from build123d import *

# Parameters (mm, degrees)
CROQUIS2_W              = 43
CROQUIS2_H              = 82
SALIENTE_EXTRUIR1_DEPTH = 24
CROQUIS3_W              = 24.22772491
CROQUIS3_H              = 79.582021813
CORTAR_EXTRUIR1_DEPTH   = 16
CROQUIS4_W              = 16.121738507
CROQUIS4_H              = 21.293525096
CORTAR_EXTRUIR2_DEPTH   = 10
CORTAR_EXTRUIR4_DEPTH   = 89.103632161
REDONDEO1_R             = 10
SALIENTE_EXTRUIR3_DEPTH = 16
CROQUIS8_W              = 4.909457408
CROQUIS8_H              = 15
SALIENTE_EXTRUIR4_DEPTH = 10
CORTAR_EXTRUIR5_START   = -4.909458
CROQUIS9_R              = 3
CORTAR_EXTRUIR5_DEPTH   = 4.909458
SALIENTE_EXTRUIR5_DEPTH = 9.5
CROQUIS12_W             = 8.494170986
CROQUIS12_H             = 20
SALIENTE_EXTRUIR6_DEPTH = 18
CROQUIS12_3_W           = 8.498446764
CROQUIS12_3_H           = 21
CORTAR_EXTRUIR6_DEPTH   = 15
CROQUIS13_W             = 4.947680971
CROQUIS13_H             = 17.318298189
CORTAR_EXTRUIR8_DEPTH   = 15
REDONDEO6_R             = 4
CROQUIS14_W             = 12
CROQUIS14_H             = 10
SALIENTE_EXTRUIR7_DEPTH = 15
CROQUIS16_R             = 3.3
CORTAR_EXTRUIR9_DEPTH   = 85.026241651
SALIENTE_EXTRUIR8_DEPTH = 10
CROQUIS21_R             = 3.3
CORTAR_EXTRUIR10_DEPTH  = 93.393365129
CROQUIS22_W             = 6
CROQUIS22_H             = 15
SALIENTE_EXTRUIR9_DEPTH = 10
CROQUIS23_R             = 3
CORTAR_EXTRUIR11_DEPTH  = 10


with BuildPart() as part:
    # Croquis2 → Saliente-Extruir1 (new body)
    with BuildSketch(Plane(origin=(0, 0, 0), x_dir=(0, 0, -1), z_dir=(1, 0, 0))):
        Rectangle(CROQUIS2_W, CROQUIS2_H)
    extrude(amount=SALIENTE_EXTRUIR1_DEPTH)

    # Croquis3 → Cortar-Extruir1 (cut)
    with BuildSketch(Plane.ZY):
        with Locations((-6.735600962, -1.208989093)):
            Rectangle(CROQUIS3_W, CROQUIS3_H)
    extrude(amount=-CORTAR_EXTRUIR1_DEPTH, mode=Mode.SUBTRACT)

    # Croquis4 → Cortar-Extruir2 (cut)
    with BuildSketch(Plane.ZY):
        with Locations((13.439130747, 15.935259265)):
            Rectangle(CROQUIS4_W, CROQUIS4_H)
    extrude(amount=-CORTAR_EXTRUIR2_DEPTH, mode=Mode.SUBTRACT)

    # Croquis5 → Cortar-Extruir4 (cut, through all)
    with BuildSketch(Plane(origin=(0, 41, 0), x_dir=(1, 0, 0), z_dir=(0, 1, 0))):
        with BuildLine():
            Line((0, 14.078023223), (0, 4.478023223))
            ThreePointArc((0, 4.478023223), (4.8, 9.278023223), (0, 14.078023223))
        make_face()
    extrude(amount=-CORTAR_EXTRUIR4_DEPTH, mode=Mode.SUBTRACT)

    # Redondeo1
    # the kernel refuses this fillet: 10 mm, written as the material it takes off along each edge
    with BuildSketch(Plane(origin=(24, 66, -21.5), x_dir=(0, 0, 1), z_dir=(0, -1, 0))) as redondeo1_piece_1:
        with BuildLine():
            CenterArc((REDONDEO1_R, REDONDEO1_R), REDONDEO1_R, 180, 90)
            Line((0, REDONDEO1_R), (0, 0))
            Line((0, 0), (REDONDEO1_R, 0))
        make_face()
    extrude(amount=132, mode=Mode.SUBTRACT)
    with BuildSketch(Plane(origin=(24, 41, 46.5), x_dir=(0, -1, 0), z_dir=(0, 0, -1))) as redondeo1_piece_2:
        with BuildLine():
            CenterArc((REDONDEO1_R, REDONDEO1_R), REDONDEO1_R, 180, 90)
            Line((0, REDONDEO1_R), (0, 0))
            Line((0, 0), (REDONDEO1_R, 0))
        make_face()
    extrude(amount=93, mode=Mode.SUBTRACT)
    with BuildSketch(Plane(origin=(24, -66, 21.5), x_dir=(-1, 0, 0), z_dir=(0, 1, 0))) as redondeo1_piece_3:
        with BuildLine():
            CenterArc((REDONDEO1_R, -REDONDEO1_R), REDONDEO1_R, 90, 90)
            Line((0, -REDONDEO1_R), (0, 0))
            Line((0, 0), (REDONDEO1_R, 0))
        make_face()
    extrude(amount=132, mode=Mode.SUBTRACT)
    with BuildSketch(Plane(origin=(24, -41, -46.5), x_dir=(-1, 0, 0), z_dir=(0, 0, 1))) as redondeo1_piece_4:
        with BuildLine():
            CenterArc((REDONDEO1_R, -REDONDEO1_R), REDONDEO1_R, 90, 90)
            Line((0, -REDONDEO1_R), (0, 0))
            Line((0, 0), (REDONDEO1_R, 0))
        make_face()
    extrude(amount=93, mode=Mode.SUBTRACT)

    # Croquis7 → Saliente-Extruir3 (add)
    with BuildSketch(Plane.XY.offset(21.5)):
        with BuildLine():
            Line((0, -41), (14, -41))
            Line((14, -41), (14, 41))
            Line((14, 41), (0, 41))
            Line((0, 41), (0, 26.582021813))
            ThreePointArc((0, 26.582021813), (10, 15.935259265), (0, 5.288496717))
            Line((0, 5.288496717), (0, -41))
        make_face()
    extrude(amount=-SALIENTE_EXTRUIR3_DEPTH)

    # Croquis8 → Saliente-Extruir4 (add)
    with BuildSketch(Plane(origin=(0, 0, -21.5), x_dir=(-1, 0, 0), z_dir=(0, 0, -1))):
        with Locations((-2.454728704, 13.5)):
            Rectangle(CROQUIS8_W, CROQUIS8_H)
        with Locations((-2.454728704, -13.5)):
            Rectangle(CROQUIS8_W, CROQUIS8_H)
    extrude(amount=SALIENTE_EXTRUIR4_DEPTH)

    # Croquis9 → Cortar-Extruir5 (cut)
    with BuildSketch(Plane(origin=(4.909457408, 0, 0), x_dir=(0, 0, -1), z_dir=(1, 0, 0)).offset(CORTAR_EXTRUIR5_START)):
        with Locations(Location((26.5, 13.5, 0), (0, 0, 90))):
            Circle(CROQUIS9_R)
        with Locations(Location((26.5, -13.5, 0), (0, 0, 90))):
            Circle(CROQUIS9_R)
    extrude(amount=CORTAR_EXTRUIR5_DEPTH, mode=Mode.SUBTRACT)

    # Croquis10 → Saliente-Extruir5 (add)
    with BuildSketch(Plane(origin=(0, -41, 0), x_dir=(-1, 0, 0), z_dir=(0, -1, 0))):
        with BuildLine():
            Line((0, -19.532438339), (0, -13.132438339))
            ThreePointArc((0, -13.132438339), (-3.2, -16.332438339), (0, -19.532438339))
        make_face()
    extrude(amount=SALIENTE_EXTRUIR5_DEPTH)

    # Croquis12 → Saliente-Extruir6 (add)
    with BuildSketch(Plane.ZY):
        with Locations((-23.09654891, -31)):
            Rectangle(CROQUIS12_W, CROQUIS12_H)
    extrude(amount=-SALIENTE_EXTRUIR6_DEPTH)

    # Croquis12<3> → Cortar-Extruir6 (cut)
    with BuildSketch(Plane.ZY):
        with Locations((9.627484875, -30.5)):
            Rectangle(CROQUIS12_3_W, CROQUIS12_3_H)
    extrude(amount=-CORTAR_EXTRUIR6_DEPTH, mode=Mode.SUBTRACT)

    # Croquis13 → Cortar-Extruir8 (cut)
    with BuildSketch(Plane.ZY):
        with Locations((-21.323303903, -32.340850905)):
            Rectangle(CROQUIS13_W, CROQUIS13_H)
    extrude(amount=-CORTAR_EXTRUIR8_DEPTH, mode=Mode.SUBTRACT)

    # Redondeo6
    redondeo6_edges = [part.edges().sort_by_distance(p)[0] for p in [
        (11.454728704, -21, -27.343634403),
        (9, -41, -27.343634403),
        (18, -31, -27.343634403),
    ]]
    fillet(redondeo6_edges, radius=REDONDEO6_R)

    # Croquis14 → Saliente-Extruir7 (add)
    with BuildSketch(Plane.XY.offset(21.5)):
        with Locations((7.059903913, -35.778543354)):
            Rectangle(CROQUIS14_W, CROQUIS14_H)
    extrude(amount=SALIENTE_EXTRUIR7_DEPTH)

    # Croquis16 → Cortar-Extruir9 (cut, through all)
    with BuildSketch(Plane(origin=(0, -30.778543354, 0), x_dir=(1, 0, 0), z_dir=(0, 1, 0))):
        with Locations(Location((7.059903913, -29, 0), (0, 0, 270))):
            Circle(CROQUIS16_R)
        with Locations((33.516786786, 28.018487534)):
            Circle(CROQUIS16_R)
    extrude(amount=-CORTAR_EXTRUIR9_DEPTH, mode=Mode.SUBTRACT)

    # Croquis19 → Saliente-Extruir8 (add)
    with BuildSketch(Plane(origin=(0, -41, 0), x_dir=(1, 0, 0), z_dir=(0, 1, 0))):
        Polygon((43.22114317, 23.806345729), (20.704482672, 10.806345729), (12.204482672, 25.528777593), (34.72114317, 38.528777593), align=None)
    extrude(amount=SALIENTE_EXTRUIR8_DEPTH)

    # Croquis21 → Cortar-Extruir10 (cut, through all)
    with BuildSketch(Plane(origin=(0, -31, 0), x_dir=(1, 0, 0), z_dir=(0, 1, 0))):
        with Locations(Location((33.516786786, 28.018487534, 0), (0, 0, 270))):
            Circle(CROQUIS21_R)
    extrude(amount=-CORTAR_EXTRUIR10_DEPTH, mode=Mode.SUBTRACT)

    # Croquis22 → Saliente-Extruir9 (add)
    with BuildSketch(Plane.XY.offset(21.5)):
        with Locations((3, -7.5)):
            Rectangle(CROQUIS22_W, CROQUIS22_H)
    extrude(amount=SALIENTE_EXTRUIR9_DEPTH)

    # Croquis23 → Cortar-Extruir11 (cut)
    with BuildSketch(Plane(origin=(6, 0, 0), x_dir=(0, 0, -1), z_dir=(1, 0, 0))):
        with Locations(Location((-26.5, -7.5, 0), (0, 0, 90))):
            Circle(CROQUIS23_R)
    extrude(amount=-CORTAR_EXTRUIR11_DEPTH, mode=Mode.SUBTRACT)


solid = part.part
For this review, take the finished solid that the model builds, in its own axes (mm). A direction names the side the tool comes from. Give positions to 0.01 mm unless a question says otherwise; leave off trailing zeros. Loops run counter-clockwise (first coordinate to the right, second up) from the corner with the lowest first, then second, coordinate; pieces in that order, holes last. Notation, with made-up numbers: (54, 0) - (79, 0) arc R26 cw to (79, 14) - close; hole circle Ø9 at (27.25, 84.25). An arc over 180 degrees is marked (long way). Write each question's results on one line, items separated by ' | '.
(1) Take a section at A-A (y = -8). Give the boundary of the cut face in (x, z).
Conclusion:
outline: (0, -31.5) - (4.91, -31.5) - (4.91, -21.5) - (14, -21.5) arc R10 ccw to (24, -11.5) - (24, 11.5) arc R10 ccw to (14, 21.5) - (6, 21.5) - (6, 23.54) - (0, 23.54) - (0, 5.38) - (16, 5.38) - (16, -18.85) - (0, -18.85) - close; (0, 29.46) - (6, 29.46) - (6, 31.5) - (0, 31.5) - close
(2) For line 1 along Z through (x, y) = (4, -7.5); line 2 along Z through (x, y) = (12, 8.5); line 3 along X through (y, z) = (-32, 29), list the stretches that pass through material, from the lowest coordinate up.
Conclusion:
line 1: -31.5 to -18.85, 5.38 to 23.5, 29.5 to 31.5 | line 2: -21.5 to -18.85, 5.38 to 21.5 | line 3: 1.06 to 3.76, 10.36 to 13.06
(3) Take a section at B-B (z = -1.5). Give the boundary of the cut face in (x, y).
Conclusion:
outline: (0, 38.58) - (16, 38.58) - (16, -40.8) arc R10 ccw to (24, -31) - (24, 31) arc R10 ccw to (14, 41) - (0, 41) - close
(4) For pin 1 Ø5.5 at (x, y) = (3.5, 12.5) entering from -Z; pin 2 Ø5 at (y, z) = (-40.5, 6) entering from +X; pin 3 Ø1 at (y, z) = (-37.5, -16) entering from -X, all flat-tipped, find the tip position at first contact; note any pin that passes through.
Conclusion:
pin 1: z = -31.5 | pin 2: x = 21.14 | pin 3: x = 16
(5) Take a section at D-D (z = 9). Give the boundary of the cut face in (x, y), then the cut area to 3 significant figures.
Conclusion:
outline: (0, -20) - (15, -20) - (15, -40.95) arc R10 ccw to (24, -31) - (24, 31) arc R10 ccw to (14, 41) - (0, 41) - (0, 26.58) arc R10.67 cw to (0, 5.29) - close | area: 1,450 mm^2
(6) Take a section at C-C (y = -27). Give the boundary of the cut face in (x, z).
Conclusion:
outline: (0, -27.34) - (14, -27.34) arc R4 ccw to (18, -23.34) - (18, -20.67) arc R10 ccw to (24, -11.5) - (24, 11.5) arc R10 ccw to (14, 21.5) - (0, 21.5) - (0, 13.88) - (15, 13.88) - (15, 5.38) - (16, 5.38) - (16, -18.85) - (15, -18.85) - (15, -23.8) - (0, -23.8) - close
(7) For faces 4 (the flat face through (3, 0, 26)), 5 (the flat face through (2, 21, -26)), 6 (the flat face through (4.909, -16, -24)), 7 (the flat face through (16, -1, -7)), 8 (the flat face through (8.3, -40.779, 25.6)), list the 3-axis set-ups (+Z, -Z, +X, -X, +Y, -Y) from which the entire face can be reached by the end or side of a thin tool; tool diameter is ignored.
Conclusion:
face 4: +Z, +X, -X, +Y | face 5: -Z, +X, -X, +Y | face 6: -Z, +X, +Y | face 7: -X, -Y | face 8: +Z, +X, -X, -Y
(8) Draft analysis for pull direction Y (two halves, no side actions). For faces 1 (the flat face through (8, 24, 5.5)), 2 (the flat face through (8, 7, -18.849)), 3 (the flat face through (1, -50.5, 16)), state which applies: +Y half, -Y half, draft (parallel to the pull), parting line (faces both ways), or undercut.
Conclusion:
face 1: undercut | face 2: draft | face 3: -Y half
